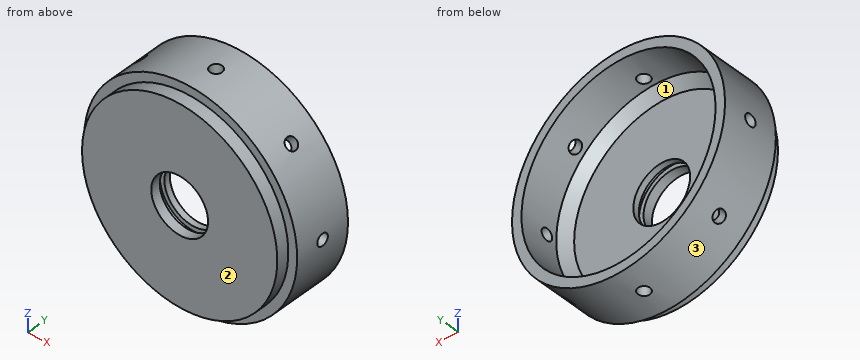
Autodesk Inventor part; units mm, degrees
ref_plane "YZ Plane" through (0, 0, 0) normal (1, 0, 0) x (0, 1, 0)
ref_plane "XZ Plane" through (0, 0, 0) normal (0, 1, 0) x (-1, 0, 0)
ref_plane "XY Plane" through (0, 0, 0) normal (0, 0, 1) x (1, 0, 0)
sketch "Sketch1" plane through (0, 0, 0) normal (0, 0, 1) x (1, 0, 0)
  line L0 (-71.4375, 45.085) -> (-65.0875, 45.085)
  line L1 (-19.05, 0) -> (-19.05, 5.08)
  line L2 (-19.05, 5.08) -> (-22.051, 5.08)
  line L3 (-22.051, 5.08) -> (-22.051, 8.6106)
  line L4 (-22.051, 8.6106) -> (-19.05, 8.6106)
  line L5 (-19.05, 0) -> (-19.05, 5.08)
  line L6 (-19.05, 8.6106) -> (-19.05, 12.7)
  line L7 (0, 0) -> (0, 17.0653)
  line L8 (-71.4375, 6.985) -> (-65.4939, 6.985)
  line L9 (-65.4939, 6.985) -> (-65.4939, 0)
  line L10 (-71.4375, 45.085) -> (-71.4375, 6.985)
  line L11 (-65.4939, 0) -> (-65.4939, -1.27)
  line L12 (-65.4939, -1.27) -> (-19.05, -1.27)
  line L13 (-19.05, -1.27) -> (-19.05, 0)
  line L14 (-65.0875, 19.05) -> (-58.7375, 12.7)
  line L15 (-65.0875, 45.085) -> (-65.0875, 19.05)
  line L16 (-58.7375, 12.7) -> (-19.05, 12.7)
  dimension "d3" = 19.05
  dimension "d8" = 12.7
  dimension "d9" = 5.08
  dimension "d10" = 3.001
  dimension "d11" = 3.5306
  dimension "d12" = 4.0894
  dimension "d26" = 5.9436
  dimension "d28" = 1.27
  dimension "d29" = 6.985
  dimension "d30" = 38.1
  dimension "d31" = 46.4439
  dimension "d32" = 1.27
  dimension "d35" = 39.6875
  dimension "d37" = 135
  dimension "d40" = 71.4375
  dimension "d41" = 20.32
  dimension "d42" = 26.035
revolve "Revolution3" add sketch "Sketch1" angle 360 about axis through (0, 0, 0) along (0, 1, 0)
sketch "Sketch2" plane through (0, 0, 0) normal (1, 0, 0) x (0, 1, 0)
  line L0 (45.085, -65.0875) -> (45.085, 65.0875)
  circle A0 centre (26.035, 0) radius 3.9688
  point P0 (0, 0)
  dimension "d45" = 7.9375
extrude "Extrusion1" cut sketch "Sketch2" along normal blind 207.9625
pattern_circular "Circular Pattern1" count 8 over 360 about axis through (0, 32.0675, 0) along (0, 1, 0) of "Extrusion1"
properties part number "Forward Closure" material "Aluminum 6061 T6 0 Cold Formed"
Input: part model. Units: mm. Frame: model coordinates. Face numbers are marked on the shaded views. Round coordinates to 2 decimals unless told otherwise and drop trailing zeros. Write each loop counter-clockwise with the first axis right and the second up, starting at its lowest first coordinate (ties: lowest second). Pieces come first, ordered by that corner, then holes.
1) Draft query along X for the marked faces 1, 2 and 3. Return one class per face: pulls with the +X half, pulls with the -X half, needs draft (parallel to the pull), parting line crosses it, or undercut.
2) Cut plane D-D (y = 3). Return the cut outline in (x, z).
3) Contact query for flat-ended pins moving along their axis: P1, Ø3, axis at y = 18, z = 18.5, coming from the +X side; P2, Ø9, axis at y = 26.035, z = 0, coming from the +X side; P3, Ø2, axis at x = -43.5, z = 46, coming from the +Y side; P4, Ø2, axis at x = -56, y = 10.5, coming from the +Z side. Output: stop coordinate, or through.
4) Cut plane C-C (y = 33). Return the cut outline in (x, z) (1 decimal), then the cut area to 3 significant figures.
5) Cut plane A-A (z = 0). Count the separate pieces of the cut face and the enclosed holes in it, then the cut area to 3 significant figures.
6) Ray query, L1, parallel to Z at x = 0, y = 2; L2, parallel to Z at x = 0, y = 33. Return the intervals inside material, ascending.
Geometry says:
1. face 1: undercut
1. face 2: needs draft
1. face 3: parting line crosses it
2. outline: circle Ø130.99 at (0, 0); hole circle Ø38.1 at (0, 0)
3. P1: stops at x = 69.39
3. P2: stops at x = 71.44
3. P3: stops at y = 18.27
3. P4: stops at z = 45.59
4. outline: circle Ø142.9 at (0, 0); hole circle Ø130.2 at (0, 0)
4. area: 2,720 mm2
5. separate pieces: 4
5. enclosed holes: 0
5. area: 1,700 mm2
6. L1: z = -65.49 to -19.05, 19.05 to 65.49
6. L2: z = -71.44 to -65.09, 65.09 to 71.44
